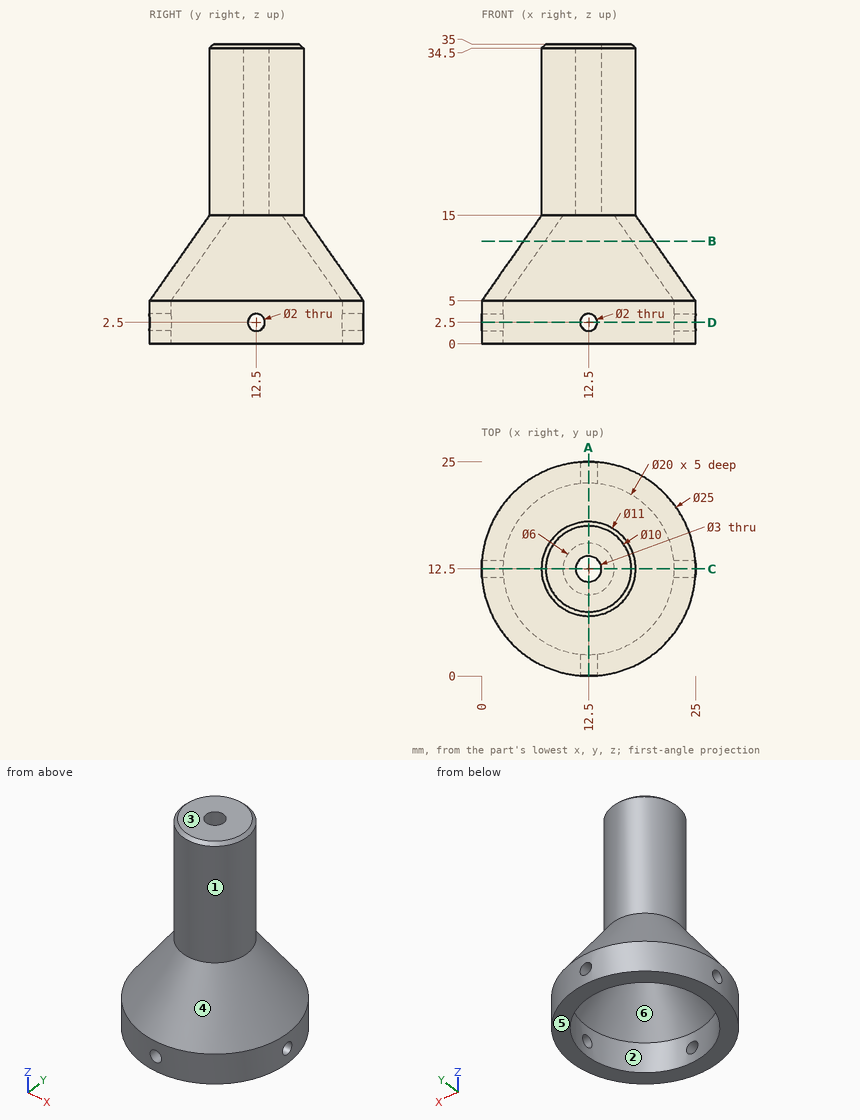
Can you work these out from the drawing? Everything is in mm from the part's minimum corner. A direction names the side the tool comes from. Coordinates: 2 decimals unless noted, no trailing zeros. Order: outer loops, then holes, each group sorted by start corner. A loop starts at its lowest first (then second) coordinate and runs counter-clockwise, first axis right, second up. Notation, with made-up numbers: (-0.5, -26) -> (3.5, -26) arc R26 ccw to (3.5, 7) -> close; hole circle Ø7 at (46.5, 68.5). An arc over 180 degrees is marked (long way). Return JSON: item names as keys, results as strings.
1) On a 3-axis mill with a long thin cutter (end or side, diameter ignored), from which of +Z, -Z, +X, -X, +Y, -Y can I reach the whole of each face in a straight line? I mean the marked faces 1, 2 and 3. Say none if no direction works.
Conclusion:
{"face 1": "+Z", "face 2": "-Z", "face 3": "+Z, +X, -X, +Y, -Y"}
2) If we section it at C-C on y = 12.5: State how many separate pieces and enclosed holes the cut face has, plus the area to 3 significant figures.
Conclusion:
{"separate pieces": "4", "enclosed holes": "0", "area": "225 mm²"}
3) If we section it at A-A on x = 12.5: List the corners of the cut face in (y, z) for me.
Conclusion:
{"outline": "(0, 0) -> (2.5, 0) -> (2.5, 1.5) -> (0, 1.5) -> close; (0, 3.5) -> (2.5, 3.5) -> (2.5, 5) -> (9.5, 15) -> (11, 15) -> (11, 35) -> (7.5, 35) -> (7, 34.5) -> (7, 15) -> (0, 5) -> close; (14, 15) -> (15.5, 15) -> (22.5, 5) -> (22.5, 3.5) -> (25, 3.5) -> (25, 5) -> (18, 15) -> (18, 34.5) -> (17.5, 35) -> (14, 35) -> close; (22.5, 0) -> (25, 0) -> (25, 1.5) -> (22.5, 1.5) -> close"}
4) If we section it at B-B on z = 12: List the corners of the cut face in (x, y) for me, plus the area to 3 significant figures.
Conclusion:
{"outline": "circle Ø15.2 at (12.5, 12.5); hole circle Ø10.2 at (12.5, 12.5)", "area": "99.7 mm²"}
5) If I drill on probe 1 along Y at (x, z) = (12.5, 3.65); probe 2 along X at (y, z) = (13, 32.5); probe 3 along Z at (x, y) = (12.5, 23.55), over which ranges is the centre line in solid material (lowest first)?
Conclusion:
{"probe 1": "y = 0 to 2.5, 22.5 to 25", "probe 2": "x = 7.02 to 11.09, 13.91 to 17.98", "probe 3": "z = 0 to 1.5, 3.5 to 7.07"}
6) If we section it at D-D on z = 2.5: List the corners of the cut face in (x, y) for me.
Conclusion:
{"outline": "(0.04, 11.5) arc R12.5 ccw to (11.5, 0.04) -> (11.5, 2.55) arc R10 cw to (2.55, 11.5) -> close; (0.04, 13.5) -> (2.55, 13.5) arc R10 cw to (11.5, 22.45) -> (11.5, 24.96) arc R12.5 ccw to start; (13.5, 0.04) arc R12.5 ccw to (24.96, 11.5) -> (22.45, 11.5) arc R10 cw to (13.5, 2.55) -> close; (13.5, 22.45) arc R10 cw to (22.45, 13.5) -> (24.96, 13.5) arc R12.5 ccw to (13.5, 24.96) -> close"}
7) I'm going to push flat-ended pins straight in: P1, Ø1.5, axis at x = 6.5, y = 10.5, coming from the -Z side; P2, Ø6.5, axis at x = 13.5, y = 12, coming from the -Z side; P3, Ø1.8, axis at x = 12.5, z = 2.5, coming from the +Y side; P4, Ø3, axis at x = 16.5, z = 20.5, coming from the -Y side. Where does each tip first touch, or does it pass through?
Conclusion:
{"P1": "stops at z = 9.18", "P2": "stops at z = 13.05", "P3": "passes through", "P4": "stops at y = 7.6"}
8) Thinking about a two-plate mould opening in X: for the marked faces 4, 5 and 6, which applies, +X half, -X half, draft (parallel to the pull), parting line (faces both ways), or undercut?
Conclusion:
{"face 4": "parting line", "face 5": "draft", "face 6": "undercut"}
